```python
from build123d import *

# Parameters (mm, degrees)
BOSS_EXTRUDE1_DEPTH = 220
SKETCH2_R           = 4.75
CUT_EXTRUDE1_DEPTH  = 8.5
SKETCH3_R           = 3
CUT_EXTRUDE2_DEPTH  = 221.391129586
LPATTERN1_COUNT     = 4
LPATTERN1_PITCH     = 60


with BuildPart() as part:
    # Sketch1 → Boss-Extrude1 (new body)
    with BuildSketch(Plane(origin=(0, 0, 0), x_dir=(0, 0, -1), z_dir=(1, 0, 0))):
        Polygon((9, 0), (-9, 0), (-10, 1), (-10, 5.5), (-8, 7), (-8, 8.5), (-10, 10.5), (-10, 13.5), (-8, 15.5), (8, 15.5), (10, 13.5), (10, 10.5), (8, 8.5), (8, 7), (10, 5.5), (10, 1), align=None)
    extrude(amount=BOSS_EXTRUDE1_DEPTH)

    # Sketch2 → Cut-Extrude1 (cut)
    with BuildSketch(Plane(origin=(0, 15.5, 0), x_dir=(1, 0, 0), z_dir=(0, 1, 0))):
        with Locations(Location((20, 0, 0), (0, 0, 270))):
            Circle(SKETCH2_R)
    cut_extrude1 = extrude(amount=-CUT_EXTRUDE1_DEPTH, mode=Mode.SUBTRACT)

    # Sketch3 → Cut-Extrude2 (cut, through all)
    with BuildSketch(Plane(origin=(0, 7, 0), x_dir=(1, 0, 0), z_dir=(0, 1, 0))):
        with Locations(Location((20, 0, 0), (0, 0, 270))):
            Circle(SKETCH3_R)
    cut_extrude2 = extrude(amount=-CUT_EXTRUDE2_DEPTH, mode=Mode.SUBTRACT)

    # LPattern1: Cut-Extrude1, Cut-Extrude2 ×4
    with Locations(*[(i * LPATTERN1_PITCH, 0, 0) for i in range(1, LPATTERN1_COUNT)]):
        add(cut_extrude1, mode=Mode.SUBTRACT)
        add(cut_extrude2, mode=Mode.SUBTRACT)


solid = part.part
```
Design review of the part built by this model. Coordinates are the model's own, in mm. A direction names the side the tool comes from. Coordinates: 2 decimals unless noted, no trailing zeros. Order: outer loops, then holes, each group sorted by start corner. A loop starts at its lowest first (then second) coordinate and runs counter-clockwise, first axis right, second up.
1) Wall thickness on line 1 along X through (y, z) = (5.5, 0); line 2 along X through (y, z) = (8.75, 0); line 3 along Z through (x, y) = (140, 1.75): over which ranges is each line inside the solid? List them lowest first.
2) Take a section at D-D, the plane x = 119. Give the boundary of the cut face in (y, z), and give its area (3 significant figures).
3) Clearance check with flat-ended pins moving along their axes: pin 1 (3 mm diameter, centred on x = 138.5, z = 0.5, fed in from +Y); pin 2 (0.8 mm diameter, centred on x = 94.5, y = 8, fed in from +Z). State where each tip first meets the part, or that it passes through.
4) Take a section at C-C, the plane z = 0. State how many separate pieces and enclosed holes the cut face has, and give its area (3 significant figures).
5) For faces 1 (the flat face through (19, 7, 3)), 2 (the flat face through (220, 8, 0)), list the 3-axis set-ups (+Z, -Z, +X, -X, +Y, -Y) from which the entire face can be reached by the end or side of a thin tool; tool diameter is ignored.
6) Take a section at A-A, the plane x = 80. Give the boundary of the cut face in (y, z).
7) Mouldability with a two-part tool opening along Z and no side actions: class faces 3 (the flat face through (0, 8, 0)), 4 (the flat face through (108, 3, 10)), 5 (the flat face through (108, 3, -10)), 6 (the cylindrical face through (17.07, 3.55, -0.65)) as +Z half, -Z half, draft (parallel to the pull), parting line (faces both ways), or undercut.
8) Take a section at B-B, the plane y = 3.5. Give the boundary of the cut face in (x, z).
Returned:
1. line 1: x = 0 to 17, 23 to 77, 83 to 137, 143 to 197, 203 to 220
1. line 2: x = 0 to 15.25, 24.75 to 75.25, 84.75 to 135.25, 144.75 to 195.25, 204.75 to 220
1. line 3: z = -10 to -3, 3 to 10
2. outline: (0, -9) - (1, -10) - (5.5, -10) - (7, -8) - (8.5, -8) - (10.5, -10) - (13.5, -10) - (15.5, -8) - (15.5, 8) - (13.5, 10) - (10.5, 10) - (8.5, 8) - (7, 8) - (5.5, 10) - (1, 10) - (0, 9) - close
2. area: 292 mm2
3. pin 1: stops at y = 7
3. pin 2: stops at z = 8
4. separate pieces: 5
4. enclosed holes: 0
4. area: 2,920 mm2
5. face 1: +Y
5. face 2: +Z, -Z, +X, +Y, -Y
6. outline: (0, -9) - (1, -10) - (5.5, -10) - (7, -8) - (8.5, -8) - (10.5, -10) - (13.5, -10) - (15.5, -8) - (15.5, -4.75) - (7, -4.75) - (7, -3) - (0, -3) - close; (0, 3) - (7, 3) - (7, 4.75) - (15.5, 4.75) - (15.5, 8) - (13.5, 10) - (10.5, 10) - (8.5, 8) - (7, 8) - (5.5, 10) - (1, 10) - (0, 9) - close
7. face 3: draft
7. face 4: +Z half
7. face 5: -Z half
7. face 6: undercut
8. outline: (0, -10) - (220, -10) - (220, 10) - (0, 10) - close; hole circle Ø6 at (20, 0); hole circle Ø6 at (80, 0); hole circle Ø6 at (140, 0); hole circle Ø6 at (200, 0)
